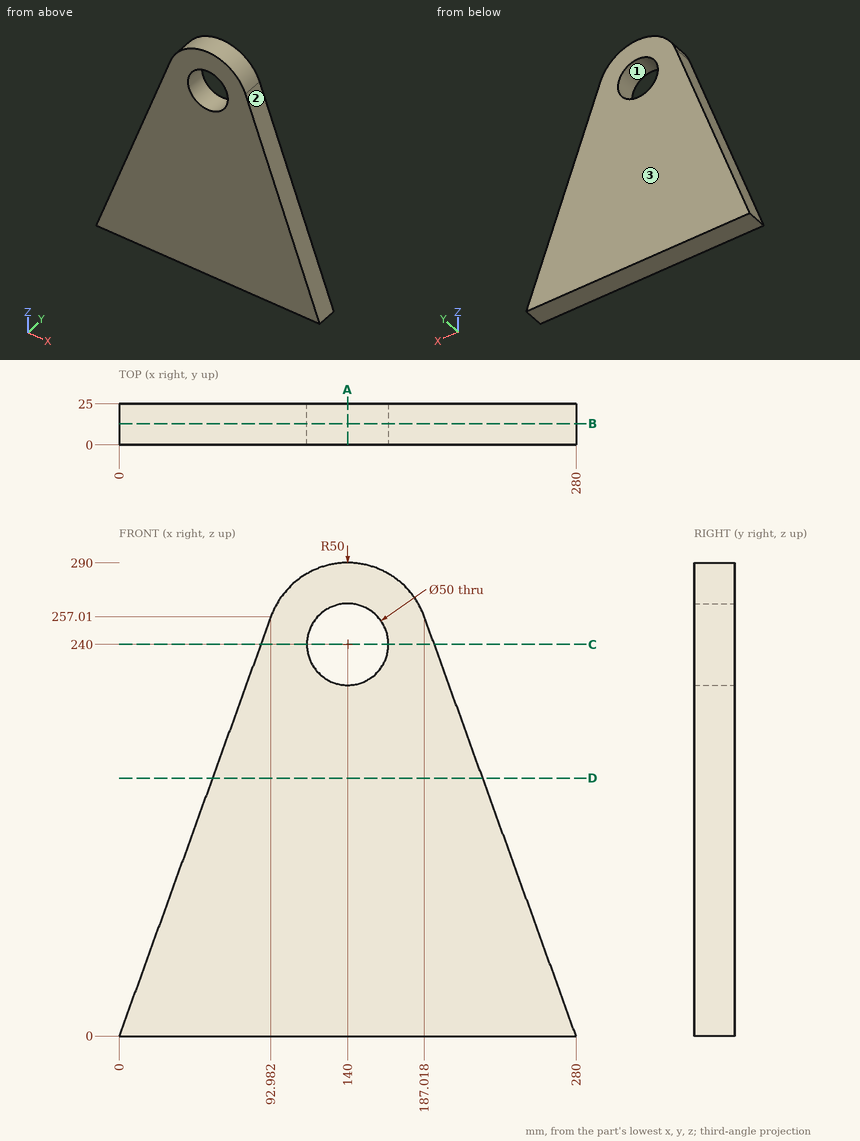
Here's the drawing with two shaded views (mm, measured from the low corner). I have some questions. Coordinates: 2 decimals unless noted, no trailing zeros. Loops run counter-clockwise (first coordinate to the right, second up) from the corner with the lowest first, then second, coordinate; pieces in that order, holes last. Notation, with made-up numbers: M 16,-31.5 L 51,-31.5 A18 ccw 51,-12.5 Z; hole C 1.25,76.25 d1. An arc over 180 degrees is marked long. Put each result on its own line as item: value. Start each with the question number.
(1) Imagine slicing it at C-C on z = 240. List the corners of the cut face in (x, y) for me.
(2) Imagine slicing it at B-B on y = 13. List the corners of the cut face in (x, z) for me, and give its area (3 significant figures).
(3) Will these pins go through, and if not, where does the flat tip stop? pin 1 Ø12 at (x, y) = (192.5, 14) entering from -Z; pin 2 Ø1.5 at (y, z) = (22, 61) entering from +X.
(4) Imagine slicing it at D-D on z = 158. List the corners of the cut face in (x, y) for me, and give its area (3 significant figures).
(5) Imagine slicing it at A-A on x = 140. List the corners of the cut face in (y, z) for me.
(6) I need wall thicknesses on probe 1 along Z at (x, y) = (140, 16.75); probe 2 along X at (y, z) = (14.75, 101.5); probe 3 along X at (y, z) = (2, 136.5) (1 decimal). Which ranges of each line are inside material? Lowest first, please.
(7) We'd pull the mould along Z, two halves only. Please class the marked faces 1, 2 and 3: +Z half, -Z half, draft (parallel to the pull), parting line (faces both ways), or undercut.
Worked answers:
1. outline: M 86.83,0 L 115,0 L 115,25 L 86.83,25 Z; M 165,0 L 193.17,0 L 193.17,25 L 165,25 Z
2. outline: M 0,0 L 280,0 L 187.02,257.01 A50 ccw 92.98,257.01 Z; hole C 140,240 d50
2. area: 48,400 mm2
3. pin 1: stops at z = 0
3. pin 2: stops at x = 258.2
4. outline: M 57.16,0 L 222.84,0 L 222.84,25 L 57.16,25 Z
4. area: 4,140 mm2
5. outline: M 0,0 L 25,0 L 25,215 L 0,215 Z; M 0,265 L 25,265 L 25,290 L 0,290 Z
6. probe 1: z = 0 to 215, 265 to 290
6. probe 2: x = 36.72 to 243.28
6. probe 3: x = 49.4 to 230.6
7. face 1: undercut
7. face 2: +Z half
7. face 3: draft
